Geometry check sheet. Reference: the model listing, model coordinates, mm. Face numbers are marked on the shaded views. A direction names the side the tool comes from. Give positions to 0.01 mm unless a question says otherwise; leave off trailing zeros. Write each loop counter-clockwise with the first axis right and the second up, starting at its lowest first coordinate (ties: lowest second). Pieces come first, ordered by that corner, then holes. Notation, with made-up numbers: M 78.25,-14.75 L 116.25,-14.75 A37 cw 116.25,22.25 Z; hole C -18.75,-36 d4. An arc over 180 degrees is marked long. One line per item, written item: value. Start each with the question number.
1. Gauge pin test, flat ends, axial feed: pin 1 (12 mm diameter, centred on y = -17.5, z = -10.5, fed in from +X); pin 2 (5 mm diameter, centred on y = -11.5, z = 19, fed in from +X); pin 3 (1.5 mm diameter, centred on y = -12.5, z = 19, fed in from +X). Record the tip position at first contact, or that the pin passes through.
2. Release check for a two-part mould opening along Z. For the marked faces 1, 2 and 3 record: pulls with the +Z half, pulls with the -Z half, needs draft (parallel to the pull), parting line crosses it, or undercut.
3. Cross-section at D-D on y = 9. Record the cut outline in (x, z), then the cut area to 3 significant figures.
4. Tool access check on the marked faces 4 and 5. Record the directions out of +Z, -Z, +X, -X, +Y, -Y that give a thin tool (end or side, any length) a straight path to the whole face; none if there is none.
5. Scan lines: line 1 (Z direction, x = 5, y = 2.5); line 2 (Y direction, x = 3.5, z = -16); line 3 (Y direction, x = 9.25, z = 5). Record each from-to range of solid material in increasing order.
6. Cross-section at B-B on z = 0.5. Record the cut outline in (x, y).
7. Cross-section at A-A on y = 13.5. Record the cut outline in (x, z), then the cut area to 3 significant figures.
8. Cross-section at C-C on x = 13.25. Record the cut outline in (y, z), then the cut area to 3 significant figures.
from build123d import *

# Parameters (mm, degrees)
SKETCH1_W           = 43
SKETCH1_H           = 55
SKETCH1_R           = 1.8
BOSS_EXTRUDE1_DEPTH = 6
BOSS_EXTRUDE2_DEPTH = 4.5
BOSS_EXTRUDE3_DEPTH = 1.6
BOSS_EXTRUDE4_DEPTH = 2
SKETCH7_R           = 3
CUT_EXTRUDE2_DEPTH  = 11
SKETCH11_W          = 25
SKETCH11_H          = 25
CUT_EXTRUDE5_DEPTH  = 11.5
SKETCH17_W          = 41.4
SKETCH17_H          = 1.2
CUT_EXTRUDE7_DEPTH  = 11


with BuildPart() as part:
    # Sketch1 → Boss-Extrude1 (new body)
    with BuildSketch(Plane.YZ):
        with Locations((-2.736471392, 0.837454611)):
            Rectangle(SKETCH1_W, SKETCH1_H)
        with Locations(Location((-11.736471392, -20.162545389, 0), (0, 0, 270))):
            Circle(SKETCH1_R, mode=Mode.SUBTRACT)
        with Locations(Location((-11.736471392, 19.837454611, 0), (0, 0, 270))):
            Circle(SKETCH1_R, mode=Mode.SUBTRACT)
        with Locations(Location((8.263528608, 19.837454611, 0), (0, 0, 270))):
            Circle(SKETCH1_R, mode=Mode.SUBTRACT)
    extrude(amount=BOSS_EXTRUDE1_DEPTH)

    # Sketch3 → Boss-Extrude2 (add)
    with BuildSketch(Plane.YZ.offset(6)):
        Polygon((-22.486471392, 25.587454611), (-22.486471392, 28.337454611), (-24.236471392, 28.337454611), (-24.236471392, -26.662545389), (18.763528608, -26.662545389), (18.763528608, 28.337454611), (17.013528608, 28.337454611), (17.013528608, 25.587454611), (17.013528608, -23.912545389), (-22.486471392, -23.912545389), align=None)
    extrude(amount=BOSS_EXTRUDE2_DEPTH)

    # Sketch5 → Boss-Extrude3 (add)
    with BuildSketch(Plane.YZ.offset(10.5)):
        Polygon((-22.936471392, 26.037454611), (-22.936471392, 28.337454611), (-24.236471392, 28.337454611), (-24.236471392, -26.662545389), (18.763528608, -26.662545389), (18.763528608, 28.337454611), (17.463528608, 28.337454611), (17.463528608, 26.037454611), (17.463528608, -24.362545389), (-22.936471392, -24.362545389), align=None)
    extrude(amount=BOSS_EXTRUDE3_DEPTH)

    # Sketch6 → Boss-Extrude4 (add)
    with BuildSketch(Plane.YZ.offset(12.1)):
        Polygon((-22.236471392, 25.337454611), (-22.236471392, 28.337454611), (-24.236471392, 28.337454611), (-24.236471392, -26.662545389), (18.763528608, -26.662545389), (18.763528608, 28.337454611), (16.763528608, 28.337454611), (16.763528608, 25.337454611), (16.763528608, -23.662545389), (-22.236471392, -23.662545389), align=None)
    extrude(amount=BOSS_EXTRUDE4_DEPTH)

    # Sketch7 → Cut-Extrude2 (cut)
    with BuildSketch(Plane.YZ.offset(14.1)):
        with Locations(Location((-11.736471392, -20.162545389, 0), (0, 0, 270))):
            Circle(SKETCH7_R)
        with Locations(Location((-11.736471392, 19.837454611, 0), (0, 0, 270))):
            Circle(SKETCH7_R)
        with Locations(Location((8.263528608, 19.837454611, 0), (0, 0, 270))):
            Circle(SKETCH7_R)
    extrude(amount=-CUT_EXTRUDE2_DEPTH, mode=Mode.SUBTRACT)

    # Sketch11 → Cut-Extrude5 (cut)
    with BuildSketch(Plane.YZ.offset(6)):
        with Locations((4.263528608, -11.162545389)):
            Rectangle(SKETCH11_W, SKETCH11_H)
    extrude(amount=-CUT_EXTRUDE5_DEPTH, mode=Mode.SUBTRACT)

    # Sketch17 → Cut-Extrude7 (cut)
    with BuildSketch(Plane.YZ.offset(14.1)):
        with Locations((-2.736471392, 26.937454611)):
            Rectangle(SKETCH17_W, SKETCH17_H)
    extrude(amount=-CUT_EXTRUDE7_DEPTH, mode=Mode.SUBTRACT)


solid = part.part
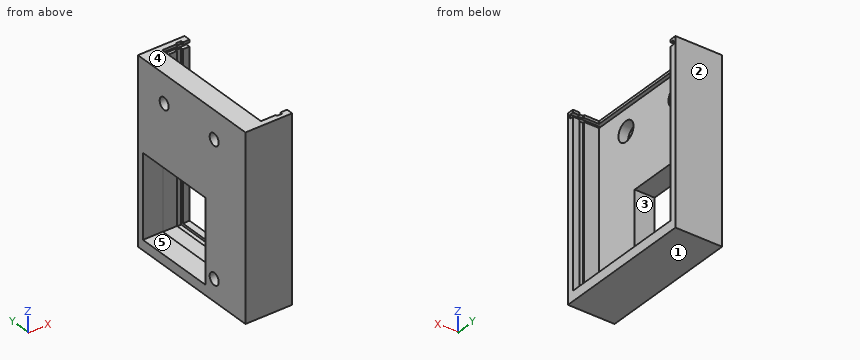
Report:
1. pin 1: stops at x = 14.1
1. pin 2: stops at x = 6
1. pin 3: stops at x = 3.1
2. face 1: pulls with the -Z half
2. face 2: needs draft
2. face 3: undercut
3. outline: M 0,-26.66 L 14.1,-26.66 L 14.1,-23.66 L 12.1,-23.66 L 12.1,-24.36 L 10.5,-24.36 L 10.5,-23.91 L 6,-23.91 L 6,-23.66 L 0,-23.66 Z; M 0,1.34 L 6,1.34 L 6,16.93 L 3.1,16.93 L 3.1,18.2 L 0,18.2 Z; M 0,21.48 L 3.1,21.48 L 3.1,22.75 L 6,22.75 L 6,26.34 L 3.1,26.34 L 3.1,27.54 L 6,27.54 L 6,28.34 L 0,28.34 Z
3. area: 172 mm^2
4. face 4: +Z, +X, -X, +Y, -Y
4. face 5: +X, -X
5. line 1: z = -26.66 to -23.66, 1.34 to 26.34, 27.54 to 28.34
5. line 2: y = -24.24 to -8.24, 16.76 to 18.76
5. line 3: y = -24.24 to -22.49, 17.01 to 18.76
6. outline: M 0,-24.24 L 14.1,-24.24 L 14.1,-22.24 L 12.1,-22.24 L 12.1,-22.94 L 10.5,-22.94 L 10.5,-22.49 L 6,-22.49 L 6,-8.24 L 0,-8.24 Z; M 0,16.76 L 6,16.76 L 6,17.01 L 10.5,17.01 L 10.5,17.46 L 12.1,17.46 L 12.1,16.76 L 14.1,16.76 L 14.1,18.76 L 0,18.76 Z
7. outline: M 0,-26.66 L 14.1,-26.66 L 14.1,-23.66 L 12.1,-23.66 L 12.1,-24.36 L 10.5,-24.36 L 10.5,-23.91 L 6,-23.91 L 6,-23.66 L 0,-23.66 Z; M 0,1.34 L 6,1.34 L 6,26.34 L 3.1,26.34 L 3.1,27.54 L 6,27.54 L 6,28.34 L 0,28.34 Z
7. area: 199 mm^2
8. outline: M -24.24,-26.66 L 18.76,-26.66 L 18.76,28.34 L 16.76,28.34 L 16.76,27.54 L 17.96,27.54 L 17.96,26.34 L 16.76,26.34 L 16.76,-23.66 L -22.24,-23.66 L -22.24,26.34 L -23.44,26.34 L -23.44,27.54 L -22.24,27.54 L -22.24,28.34 L -24.24,28.34 Z
8. area: 334 mm^2
